```python
from build123d import *

# Parameters (mm, degrees)
PAD038_DEPTH               = 3
PAD038_MIRRORED044_2_DEPTH = 3
POLARPATTERN012_COUNT      = 3
SKETCH179_R                = 15
POCKET144_DEPTH            = 5


with BuildPart() as part:
    # Sketch180 → Pad038 (new body)
    with BuildSketch(Plane.XY):
        with BuildLine():
            Line((14.3, 317.6), (14.3, 381.5))
            ThreePointArc((14.3, 381.5), (13.567767, 383.267767), (11.8, 384))
            Line((11.8, 384), (0, 384))
            Line((0, 384), (0, 0))
            Line((0, 0), (88.487966, 51.088551))
            ThreePointArc((14.3, 317.6), (33.193003, 179.277725), (88.487966, 51.088551))
        make_face()
    pad038 = extrude(amount=PAD038_DEPTH)

    # Sketch180 Mirrored044 2 → Pad038 Mirrored044 2 (add)
    with BuildSketch(Plane(origin=(0, 0, 0), x_dir=(-1, 0, 0), z_dir=(0, 0, -1))):
        with BuildLine():
            Line((14.3, 317.6), (14.3, 381.5))
            ThreePointArc((14.3, 381.5), (13.567767, 383.267767), (11.8, 384))
            Line((11.8, 384), (0, 384))
            Line((0, 384), (0, 0))
            Line((0, 0), (88.487966, 51.088551))
            ThreePointArc((14.3, 317.6), (33.193003, 179.277725), (88.487966, 51.088551))
        make_face()
    pad038_mirrored044_2 = extrude(amount=-PAD038_MIRRORED044_2_DEPTH)

    # PolarPattern012: Pad038, Pad038 Mirrored044 2 ×3 about axis
    polarpattern012_axis = Axis((0, 0, 0), (0, 0, 1))
    for i in range(1, POLARPATTERN012_COUNT):
        add(pad038.rotate(polarpattern012_axis, i * 360 / POLARPATTERN012_COUNT))
        add(pad038_mirrored044_2.rotate(polarpattern012_axis, i * 360 / POLARPATTERN012_COUNT))

    # Sketch179 → Pocket144 (cut)
    with BuildSketch(Plane.XY):
        with Locations((129.903811, -75)):
            Circle(SKETCH179_R)
        with Locations((-129.903811, -75)):
            Circle(SKETCH179_R)
    extrude(amount=POCKET144_DEPTH, mode=Mode.SUBTRACT)


solid = part.part
```
Work out the finished part from the listing and answer in its coordinate system (mm). A direction names the side the tool comes from. Coordinates: 2 decimals unless noted, no trailing zeros. Write each loop counter-clockwise with the first axis right and the second up, starting at its lowest first coordinate (ties: lowest second). Pieces come first, ordered by that corner, then holes.
Q1. Each of these flat-tipped pins is pushed along its axis until it touches: pin 1 Ø1.5 at (y, z) = (343.5, 1) entering from +X; pin 2 Ø6 at (x, y) = (72, 13.5) entering from -Z; pin 3 Ø0.9 at (y, z) = (345, 2) entering from -X; pin 4 Ø18 at (x, y) = (129.9, -75) entering from -Z. Where does it stop, or does it pass through?
Q2. A cutting plane is placed at B-B, the plane z = 0.6. Give the vertices of the cut face in (x, y), then the cut area to 3 significant figures.
Q3. A cutting plane is placed at A-A, the plane y = -75. Give the vertices of the cut face in (x, z).
Q4. Find the intervals of material crossed by line 1 (X direction, y = -75, z = 2.1); line 2 (X direction, y = -76, z = 1.4); line 3 (Y direction, x = -134, z = 2.95), in increasing order.
Q5. Which of the six approach directions +Z, -Z, +X, -X, +Y, -Y give full straight-line access (tool end or side, diameter ignored) to faces 1 (the face through (-140.56, -118.877, 1.479)), 2 (the face through (-173.23, -62.29, 1.48))?
Q6. Determine the mould class of faces 3 (the face through (-141.807, -84.127, 1.479)), 4 (the face through (140.56, -118.877, 1.479)), 5 (the face through (-309.482, -162.167, 1.479)) for opening direction Y: released by +Y, released by -Y, zero draft, split by the parting line, or undercut.
Q7. A cutting plane is placed at C-C, the plane x = -131. Give the vertices of the cut face in (y, z).
Q8. A cutting plane is placed at D-D, the plane x = 223.5. Give the vertices of the cut face in (y, z), then the cut area to 3 significant figures.
Findings below:
1. pin 1: stops at x = 14.3
1. pin 2: stops at z = 0
1. pin 3: stops at x = -14.3
1. pin 4: passes through
2. outline: (-338.45, -181.78) - (-326.65, -202.22) arc R2.5 ccw to (-323.24, -203.13) - (-267.9, -171.18) arc R515.8 cw to (0, -102.18) arc R515.8 cw to (267.9, -171.18) - (323.24, -203.13) arc R2.5 ccw to (326.65, -202.22) - (338.45, -181.78) arc R2.5 ccw to (337.54, -178.37) - (282.2, -146.42) arc R515.8 cw to (88.49, 51.09) arc R515.8 cw to (14.3, 317.6) - (14.3, 381.5) arc R2.5 ccw to (11.8, 384) - (-11.8, 384) arc R2.5 ccw to (-14.3, 381.5) - (-14.3, 317.6) arc R515.8 cw to (-88.49, 51.09) arc R515.8 cw to (-282.2, -146.42) - (-337.54, -178.37) arc R2.5 ccw to start; hole circle Ø30 at (-129.9, -75); hole circle Ø30 at (129.9, -75)
2. area: 79,000 mm2
3. outline: (-186.24, 0) - (-144.9, 0) - (-144.9, 3) - (-186.24, 3) - close; (-114.9, 0) - (114.9, 0) - (114.9, 3) - (-114.9, 3) - close; (144.9, 0) - (186.24, 0) - (186.24, 3) - (144.9, 3) - close
4. line 1: x = -186.24 to -144.9, -114.9 to 114.9, 144.9 to 186.24
4. line 2: x = -187.31 to -144.87, -114.94 to 114.94, 144.87 to 187.31
4. line 3: y = -117.21 to -89.43, -60.57 to -17.73
5. face 1: +Z, -Z, -Y
5. face 2: +Z, -Z, -X, +Y
6. face 3: undercut
6. face 4: released by -Y
6. face 5: released by +Y
7. outline: (-116.47, 0) - (-89.96, 0) - (-89.96, 3) - (-116.47, 3) - close; (-60.04, 0) - (-13.86, 0) - (-13.86, 3) - (-60.04, 3) - close
8. outline: (-148.34, 0) - (-106.92, 0) - (-106.92, 3) - (-148.34, 3) - close
8. area: 124 mm2
